Geometry: final body of the model. Coordinates: model frame, mm. A direction names the side the tool comes from. Coordinates: 2 decimals unless noted, no trailing zeros. Order: outer loops, then holes, each group sorted by start corner. A loop starts at its lowest first (then second) coordinate and runs counter-clockwise, first axis right, second up. Notation, with made-up numbers: M -1,-12.5 L 54,-12.5 A5 ccw 54,-5.5 Z; hole C 12.25,61.5 d1. An arc over 180 degrees is marked long. Write item = value, one per line. Start each with the question number.
```python
from build123d import *

# Parameters (mm, degrees)
SKETCH1_W           = 25.4
SKETCH1_H           = 25.4
SKETCH1_W_2         = 23.6
SKETCH1_H_2         = 23.6
BOSS_EXTRUDE1_DEPTH = 300
SKETCH2_R           = 7.5
CUT_EXTRUDE1_DEPTH  = 25.4
SKETCH3_R           = 3
CUT_EXTRUDE2_DEPTH  = 25.4
SKETCH4_R           = 1.5
CUT_EXTRUDE3_DEPTH  = 25.4
SKETCH5_R           = 1.5
CUT_EXTRUDE4_DEPTH  = 25.4


with BuildPart() as part:
    # Sketch1 → Boss-Extrude1 (new body)
    with BuildSketch(Plane(origin=(0, 0, 0), x_dir=(1, 0, 0), z_dir=(0, 1, 0))):
        Rectangle(SKETCH1_W, SKETCH1_H)
        Rectangle(SKETCH1_W_2, SKETCH1_H_2, mode=Mode.SUBTRACT)
    extrude(amount=BOSS_EXTRUDE1_DEPTH)

    # Sketch2 → Cut-Extrude1 (cut)
    with BuildSketch(Plane(origin=(0, 0, -12.7), x_dir=(-1, 0, 0), z_dir=(0, 0, -1))):
        with Locations((0, 20)):
            Circle(SKETCH2_R)
    extrude(amount=-CUT_EXTRUDE1_DEPTH, mode=Mode.SUBTRACT)

    # Sketch3 → Cut-Extrude2 (cut)
    with BuildSketch(Plane(origin=(0, 0, -12.7), x_dir=(-1, 0, 0), z_dir=(0, 0, -1))):
        with Locations((0, 168)):
            Circle(SKETCH3_R)
        with Locations((0, 248)):
            Circle(SKETCH3_R)
    extrude(amount=-CUT_EXTRUDE2_DEPTH, mode=Mode.SUBTRACT)

    # Sketch4 → Cut-Extrude3 (cut)
    with BuildSketch(Plane(origin=(0, 0, -12.7), x_dir=(-1, 0, 0), z_dir=(0, 0, -1))):
        with Locations((8, 9)):
            Circle(SKETCH4_R)
        with Locations((8, 31)):
            Circle(SKETCH4_R)
        with Locations((-8, 9)):
            Circle(SKETCH4_R)
        with Locations((-8, 31)):
            Circle(SKETCH4_R)
    extrude(amount=-CUT_EXTRUDE3_DEPTH, mode=Mode.SUBTRACT)

    # Sketch5 → Cut-Extrude4 (cut)
    with BuildSketch(Plane(origin=(0, 0, -12.7), x_dir=(-1, 0, 0), z_dir=(0, 0, -1))):
        with Locations((0, 220)):
            Circle(SKETCH5_R)
        with Locations((0, 265)):
            Circle(SKETCH5_R)
    extrude(amount=-CUT_EXTRUDE4_DEPTH, mode=Mode.SUBTRACT)


solid = part.part
```
Item 1: Section query C-C on y = 215.5. Output: boundary loops of the cut face in (x, z), and give its area (3 significant figures).
Item 2: Section query B-B on y = 20. Output: boundary loops of the cut face in (x, z).
Item 3: Draft query along X for faces 3 (the flat face through (0, 148, 11.8)), 4 (the flat face through (12.7, 148, 0)), 5 (the cylindrical face through (0, 251, -12)), 6 (the flat face through (-1, 300, 12)). Return one class per face: pulls with the +X half, pulls with the -X half, needs draft (parallel to the pull), parting line crosses it, or undercut.
Item 4: Reachability of faces 1 (the cylindrical face through (0, 171, 12)), 2 (the flat face through (11.8, 148, 0)) from +Z, -Z, +X, -X, +Y, -Y: full face, straight path, thin tool, end or side. Return the list, or none.
Item 5: Material intervals for probe 1 along Y at (x, z) = (8, 12.5); probe 2 along Y at (x, z) = (0, -12.45); probe 3 along X at (y, z) = (212, -7.75), sorted ascending. Write a range as [from, to].
Item 6: Section query D-D on y = 248. Output: boundary loops of the cut face in (x, z).
Item 7: First-contact query: pin 1 (2.5 mm diameter, centred on x = 8, y = 31, fed in from -Z). Flat tip, straight axial feed; report the tip coordinate or a pass-through.
Item 8: Section query A-A on z = -2.75. Output: boundary loops of the cut face in (x, y), and give its area (3 significant figures).
Ans:
q1.outline = M -12.7,-12.7 L 12.7,-12.7 L 12.7,12.7 L -12.7,12.7 Z; hole M -11.8,-11.8 L 11.8,-11.8 L 11.8,11.8 L -11.8,11.8 Z
q1.area = 88.2 mm^2
q2.outline = M -12.7,-12.7 L -7.5,-12.7 L -7.5,-11.8 L -11.8,-11.8 L -11.8,11.8 L -7.5,11.8 L -7.5,12.7 L -12.7,12.7 Z; M 7.5,-12.7 L 12.7,-12.7 L 12.7,12.7 L 7.5,12.7 L 7.5,11.8 L 11.8,11.8 L 11.8,-11.8 L 7.5,-11.8 Z
q3.face_3 = undercut
q3.face_4 = pulls with the +X half
q3.face_5 = undercut
q3.face_6 = needs draft
q4.face_1 = +Z, -Z
q4.face_2 = +Y, -Y
q5.probe_1 = [0, 7.5], [10.5, 29.5], [32.5, 300]
q5.probe_2 = [0, 12.5], [27.5, 165], [171, 218.5], [221.5, 245], [251, 263.5], [266.5, 300]
q5.probe_3 = [-12.7, -11.8], [11.8, 12.7]
q6.outline = M -12.7,-12.7 L -3,-12.7 L -3,-11.8 L -11.8,-11.8 L -11.8,11.8 L -3,11.8 L -3,12.7 L -12.7,12.7 Z; M 3,-12.7 L 12.7,-12.7 L 12.7,12.7 L 3,12.7 L 3,11.8 L 11.8,11.8 L 11.8,-11.8 L 3,-11.8 Z
q7.pin_1 = through
q8.outline = M -12.7,0 L -11.8,0 L -11.8,300 L -12.7,300 Z; M 11.8,0 L 12.7,0 L 12.7,300 L 11.8,300 Z
q8.area = 540 mm^2
